```python
from build123d import *

# Parameters (mm, degrees)
SKETCH_1_R      = 12.4
EXTRUDE_1_DEPTH = 63
SKETCH_2_R      = 3.5
EXTRUDE_2_DEPTH = 2.5
EXTRUDE_3_DEPTH = 9.68


with BuildPart() as part:
    # 草图1 → 凸台-拉伸1 (new body)
    with BuildSketch(Plane.XY):
        Circle(SKETCH_1_R)
    extrude(amount=EXTRUDE_1_DEPTH)

    # 草图2 → 凸台-拉伸2 (add)
    with BuildSketch(Plane.XY.offset(63)):
        Circle(SKETCH_2_R)
    extrude(amount=EXTRUDE_2_DEPTH)

    # 草图3 → 凸台-拉伸3 (add)
    with BuildSketch(Plane.XY.offset(65.5)):
        with BuildLine():
            Line((-1.41, 1.418414608), (-1.41, -1.418414608))
            ThreePointArc((-1.41, -1.418414608), (2, 0), (-1.41, 1.418414608))
        make_face()
    extrude(amount=EXTRUDE_3_DEPTH)


solid = part.part
```
Here's how the part is built. I have some questions about the finished solid (model axes, mm). A direction names the side the tool comes from. Coordinates: 2 decimals unless noted, no trailing zeros. Loops run counter-clockwise (first coordinate to the right, second up) from the corner with the lowest first, then second, coordinate; pieces in that order, holes last. Notation, with made-up numbers: (53, 69) - (105, 69) arc R19 cw to (105, 79) - close; hole circle Ø5 at (1, 47.5). An arc over 180 degrees is marked (long way). Answer as CSV lines item,"result".
Q1. If we section it at D-D, the plane z = 41: Write out the boundary of the cut face in (x, y), and give its area (3 significant figures).
Response:
outline,"circle Ø24.8 at (0, 0)"
area,"483 mm2"
Q2. If we section it at B-B, the plane x = 0: Write out the boundary of the cut face in (y, z).
Response:
outline,"(-12.4, 0) - (12.4, 0) - (12.4, 63) - (3.5, 63) - (3.5, 65.5) - (2, 65.5) - (2, 75.18) - (-2, 75.18) - (-2, 65.5) - (-3.5, 65.5) - (-3.5, 63) - (-12.4, 63) - close"
Q3. For faces 1 (the face through (-2, 0, 65.5)), 2 (the face through (5.72, -11, 31.06)), 3 (the face through (-1.41, 0, 70)), which set-ups out of +Z, -Z, +X, -X, +Y, -Y let a thin tool reach every point of the face, with its end or its side?
Response:
face 1,"+Z"
face 2,"+Z, -Z"
face 3,"+Z, -X, +Y, -Y"
Q4. If we section it at C-C, the plane z = 70.5: Write out the boundary of the cut face in (x, y).
Response:
outline,"(-1.41, -1.42) arc R2 ccw (long way) to (-1.41, 1.42) - close"
Q5. For pin 1 (2.5 mm diameter, centred on y = 0, z = 69, fed in from -X); pin 2 (1.5 mm diameter, centred on x = -10, y = -9, fed in from -Z); pin 3 (5 mm diameter, centred on x = -4, z = 11.5, fed in from +Y); pin 4 (3 mm diameter, centred on x = 6.5, z = 47.5, fed in from -Y), each with a flat end and sliding along its axis, tell me the tip position at first contact or that it passes through.
Response:
pin 1,"x = -1.41"
pin 2,"through"
pin 3,"y = 12.31"
pin 4,"y = -11.35"
Q6. If I drill on L1, parallel to Z at x = -1.75, y = -2; L2, parallel to Z at x = -3.5, y = 3; L3, parallel to Y at x = -1.5, z = 35, over which ranges is the centre line in solid material (lowest first)? Write a range as [from, to].
Response:
L1,"[0, 65.5]"
L2,"[0, 63]"
L3,"[-12.31, 12.31]"
Q7. If we section it at A-A, the plane y = 0: Write out the boundary of the cut face in (x, z).
Response:
outline,"(-12.4, 0) - (12.4, 0) - (12.4, 63) - (3.5, 63) - (3.5, 65.5) - (2, 65.5) - (2, 75.18) - (-1.41, 75.18) - (-1.41, 65.5) - (-3.5, 65.5) - (-3.5, 63) - (-12.4, 63) - close"
